Geometry check sheet. Reference: the model listing, model coordinates, mm. Face numbers are marked on the shaded views. A direction names the side the tool comes from. Give positions to 0.01 mm unless a question says otherwise; leave off trailing zeros. Order: outer loops, then holes, each group sorted by start corner. A loop starts at its lowest first (then second) coordinate and runs counter-clockwise, first axis right, second up. Notation, with made-up numbers: (-24.5, -25.5) - (-16.5, -25.5) arc R7 ccw to (-16.5, -12.5) - close; hole circle Ø2 at (-15, -32.75). An arc over 180 degrees is marked (long way). Put each result on its own line as item: value. Start each with the question number.
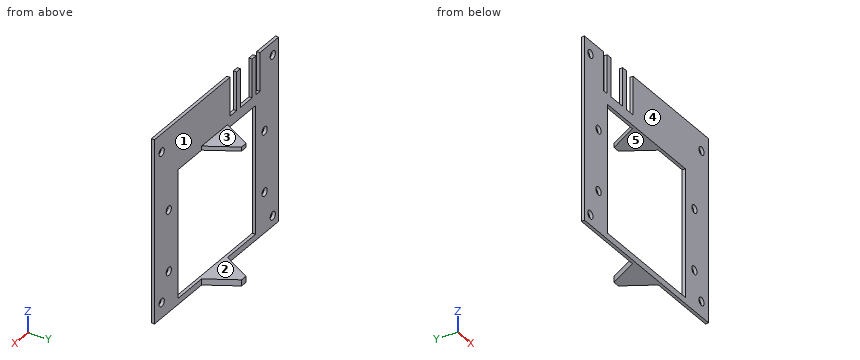
```python
from build123d import *

# Parameters (mm, degrees)
SKETCH1_W               = 96.89
SKETCH1_H               = 90.17
PCB_DEPTH               = 1.57
SKETCH2_R               = 2
M3_MOUNTING_HOLES_DEPTH = 1.57
SKETCH4_R               = 2
CUT_EXTRUDE1_DEPTH      = 23
BOSS_EXTRUDE2_DEPTH     = 2
BOSS_EXTRUDE3_DEPTH     = 3
SKETCH9_W               = 3
SKETCH9_H               = 19
SKETCH9_W_2             = 9
SKETCH9_W_3             = 5
CUT_EXTRUDE2_DEPTH      = 2.57
SKETCH10_W              = 0.5
SKETCH10_H              = 90.17
CUT_EXTRUDE3_DEPTH      = 10
SKETCH11_W              = 60
SKETCH11_H              = 63
CUT_EXTRUDE4_DEPTH      = 10


with BuildPart() as part:
    # Sketch1 → PCB (new body)
    with BuildSketch(Plane(origin=(0, 0, 0), x_dir=(1, 0, 0), z_dir=(0, 1, 0))):
        with Locations((16.200949951, 63.633996534)):
            Rectangle(SKETCH1_W, SKETCH1_H)
    extrude(amount=PCB_DEPTH)

    # Sketch2 → M3 Mounting Holes (cut)
    with BuildSketch(Plane(origin=(0, 1.57, 0), x_dir=(1, 0, 0), z_dir=(0, 1, 0))):
        with Locations((58.565949951, 27.438996534)):
            Circle(SKETCH2_R)
        with Locations((-27.164050049, 24.898996534)):
            Circle(SKETCH2_R)
        with Locations((-27.164050049, 103.638996534)):
            Circle(SKETCH2_R)
        with Locations((58.565949951, 101.098996534)):
            Circle(SKETCH2_R)
    extrude(amount=-M3_MOUNTING_HOLES_DEPTH, mode=Mode.SUBTRACT)

    # Sketch4 → Cut-Extrude1 (cut)
    with BuildSketch(Plane(origin=(0, 1.57, 0), x_dir=(1, 0, 0), z_dir=(0, 1, 0))):
        with Locations((-20.894050049, 88.718996534)):
            Circle(SKETCH4_R)
        with Locations((53.105949951, 88.718996534)):
            Circle(SKETCH4_R)
        with Locations((-20.894050049, 58.718996534)):
            Circle(SKETCH4_R)
        with Locations((53.105949951, 58.718996534)):
            Circle(SKETCH4_R)
    extrude(amount=-CUT_EXTRUDE1_DEPTH, mode=Mode.SUBTRACT)

    # Sketch7 → Boss-Extrude2 (add)
    with BuildSketch(Plane.XY.offset(-42.718996534)):
        Polygon((27.755949951, 1.57), (19.438412086, 15.976398176), (16.073487816, 15.976398176), (7.755949951, 1.57), align=None)
    extrude(amount=BOSS_EXTRUDE2_DEPTH)

    # Sketch8 → Boss-Extrude3 (add)
    with BuildSketch(Plane.XY.offset(-108.718996534)):
        Polygon((27.755949951, 1.57), (19.438412086, 15.976398176), (16.073487816, 15.976398176), (7.755949951, 1.57), align=None)
    extrude(amount=BOSS_EXTRUDE3_DEPTH)

    # Sketch9 → Cut-Extrude2 (cut, through all)
    with BuildSketch(Plane(origin=(0, 1.57, 0), x_dir=(1, 0, 0), z_dir=(0, 1, 0))):
        with Locations((-15.744050049, 28.048996534)):
            Rectangle(SKETCH9_W, SKETCH9_H)
        with Locations((-6.744050049, 28.048996534)):
            Rectangle(SKETCH9_W_2, SKETCH9_H)
        with Locations((3.255949951, 28.048996534)):
            Rectangle(SKETCH9_W_3, SKETCH9_H)
    extrude(amount=-CUT_EXTRUDE2_DEPTH, mode=Mode.SUBTRACT)

    # Sketch10 → Cut-Extrude3 (cut)
    with BuildSketch(Plane(origin=(0, 1.57, 0), x_dir=(1, 0, 0), z_dir=(0, 1, 0))):
        with Locations((-31.994050049, 63.633996534)):
            Rectangle(SKETCH10_W, SKETCH10_H)
        with Locations((64.395949951, 63.633996534)):
            Rectangle(SKETCH10_W, SKETCH10_H)
    extrude(amount=-CUT_EXTRUDE3_DEPTH, mode=Mode.SUBTRACT)

    # Sketch11 → Cut-Extrude4 (cut)
    with BuildSketch(Plane(origin=(0, 1.57, 0), x_dir=(1, 0, 0), z_dir=(0, 1, 0))):
        with Locations((16.105949951, 74.218996534)):
            Rectangle(SKETCH11_W, SKETCH11_H)
    extrude(amount=-CUT_EXTRUDE4_DEPTH, mode=Mode.SUBTRACT)


solid = part.part
```
Item 1: Cross-section at A-A (z = -82.5). Enter the section's corners in (x, y), and give its area (3 significant figures).
Item 2: Set-up check for the marked faces 3, 4 and 5: record each of +Z, -Z, +X, -X, +Y, -Y from which the full face is reachable in a straight line by a thin tool's end or side.
Item 3: Cross-section at C-C (y = 11.5). Enter the section's corners in (x, z), and give its area (3 significant figures).
Item 4: Release check for a two-part mould opening along X. For the marked faces 1 and 2 record: +X half, -X half, draft (parallel to the pull), parting line (faces both ways), or undercut.
Item 5: Cross-section at B-B (x = 18). Enter the section's corners in (y, z), and give its area (3 significant figures).
Item 6: Cross-section at D-D (z = -31). Enter the section's corners in (x, y).
Item 7: Gauge pin test, flat end, axial feed: pin 1 Ø1.3 at (x, y) = (-16, 0.5) entering from +Z. Record the tip position at first contact, or that the pin passes through.
Item 8: Thickness scan on line 1 along Z through (x, y) = (13.5, 8); line 2 along Y through (x, z) = (53.5, -76). Record the ranges inside material, lowest first.
Recorded:
1. outline: (-31.74, 0) - (-13.89, 0) - (-13.89, 1.57) - (-31.74, 1.57) - close; (46.11, 0) - (64.15, 0) - (64.15, 1.57) - (46.11, 1.57) - close
1. area: 56.3 mm^2
2. face 3: +Z, +X, -X, +Y
2. face 4: +Z, -Z, +X, -X, -Y
2. face 5: +Y, -Y
3. outline: (13.49, -108.72) - (22.02, -108.72) - (22.02, -105.72) - (13.49, -105.72) - close; (13.49, -42.72) - (22.02, -42.72) - (22.02, -40.72) - (13.49, -40.72) - close
3. area: 42.7 mm^2
4. face 1: draft
4. face 2: undercut
5. outline: (0, -108.72) - (15.98, -108.72) - (15.98, -105.72) - (0, -105.72) - close; (0, -42.72) - (15.98, -42.72) - (15.98, -40.72) - (1.57, -40.72) - (1.57, -18.55) - (0, -18.55) - close
5. area: 115 mm^2
6. outline: (-31.74, 0) - (-17.24, 0) - (-17.24, 1.57) - (-31.74, 1.57) - close; (-14.24, 0) - (-11.24, 0) - (-11.24, 1.57) - (-14.24, 1.57) - close; (-2.24, 0) - (0.76, 0) - (0.76, 1.57) - (-2.24, 1.57) - close; (5.76, 0) - (64.15, 0) - (64.15, 1.57) - (5.76, 1.57) - close
7. pin 1: stops at z = -37.55
8. line 1: z = -108.72 to -105.72, -42.72 to -40.72
8. line 2: y = 0 to 1.57
